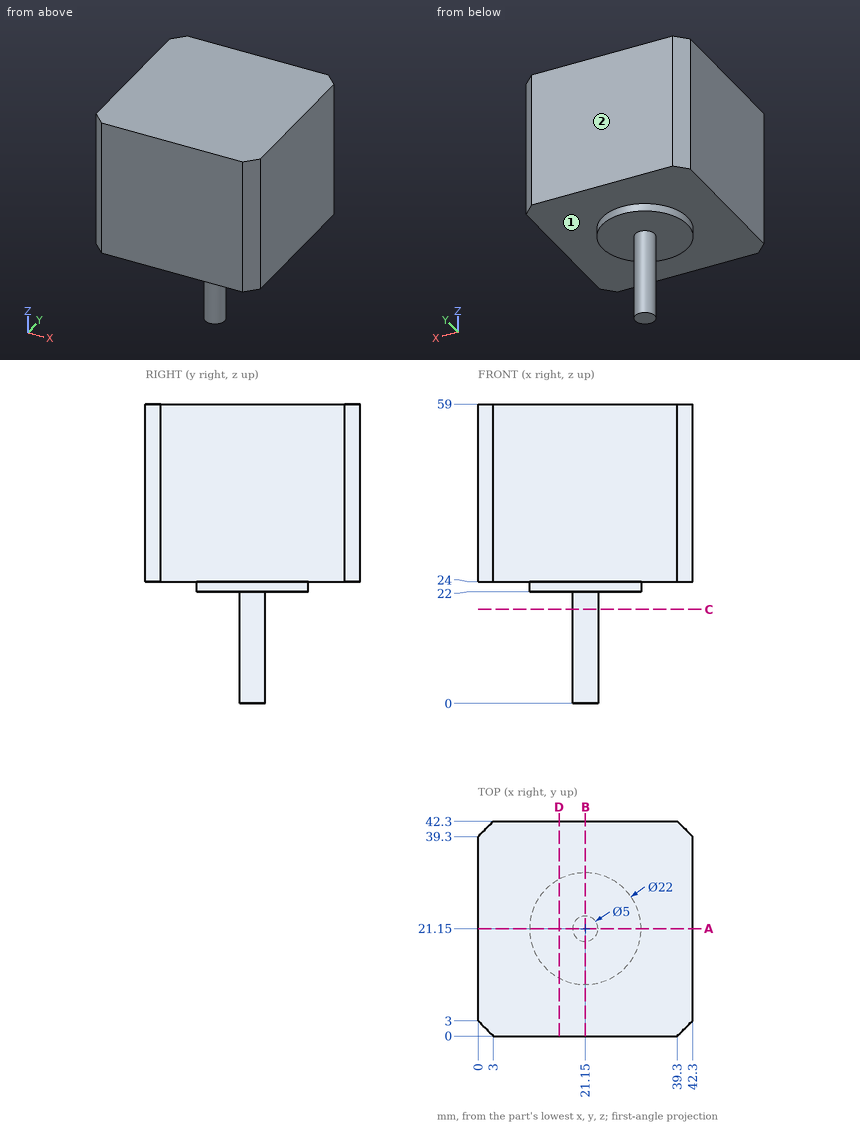
Geometry: see drawing. Coordinates: mm, zero at the bounding-box minimum. A direction names the side the tool comes from. Round coordinates to 2 decimals unless told otherwise and drop trailing zeros. Loops run counter-clockwise (first coordinate to the right, second up) from the corner with the lowest first, then second, coordinate; pieces in that order, holes last. Notation, with made-up numbers: (32, 36) -> (75, 36) arc R20 cw to (75, 53) -> close; hole circle Ø6 at (39, -1). An arc over 180 degrees is marked (long way). Write each question's results on one line, items separated by ' | '.
Item 1: Cut plane A-A on y = 21.15. Return the cut outline in (x, z), and give its area (3 significant figures).
Answers below:
outline: (0, 24) -> (10.15, 24) -> (10.15, 22) -> (18.65, 22) -> (18.65, 0) -> (23.65, 0) -> (23.65, 22) -> (32.15, 22) -> (32.15, 24) -> (42.3, 24) -> (42.3, 59) -> (0, 59) -> close | area: 1,630 mm²
Item 2: Line query: probe 1 along Z at (x, y) = (7, 24.5); probe 2 along Z at (x, y) = (21, 25.5); probe 3 along Y at (x, z) = (22, 10.5). Output: solid intervals per line, ascending. Write a range as [from, to].
Answers below:
probe 1: z = [24, 59] | probe 2: z = [22, 59] | probe 3: y = [18.8, 23.5]
Item 3: Cut plane D-D on x = 16. Return the cut outline in (y, z).
Answers below:
outline: (0, 24) -> (11.43, 24) -> (11.43, 22) -> (30.87, 22) -> (30.87, 24) -> (42.3, 24) -> (42.3, 59) -> (0, 59) -> close
Item 4: Pin query (flat end, axial travel): pin 1 Ø1.5 at (y, z) = (27, 23) entering from -X; pin 2 Ø8 at (x, z) = (15, 16.5) entering from -Y. Return the tip coordinate at first contact, or that it passes through.
Answers below:
pin 1: stops at x = 11.4 | pin 2: stops at y = 19.87
Item 5: Set-up query: the marked faces 1 and 2. Return all of +Z, -Z, +X, -X, +Y, -Y with unobstructed straight access to the full face (end or side cutting, diameter ignored); none if empty.
Answers below:
face 1: -Z | face 2: +Z, -Z, +X, -X, +Y
Item 6: Cut plane C-C on z = 18.5. Return the cut outline in (x, y).
Answers below:
outline: circle Ø5 at (21.15, 21.15)
